Verification items for this drawing (mm, ordinates from the low corner). Round coordinates to 2 decimals unless told otherwise and drop trailing zeros. Loops run counter-clockwise (first coordinate to the right, second up) from the corner with the lowest first, then second, coordinate; pieces in that order, holes last. Notation, with made-up numbers: (-11, 40.5) - (22, 40.5) arc R12 cw to (22, 48.5) - close; hole circle Ø10 at (-20.75, 66). An arc over 180 degrees is marked (long way). Write item = value, one per line.
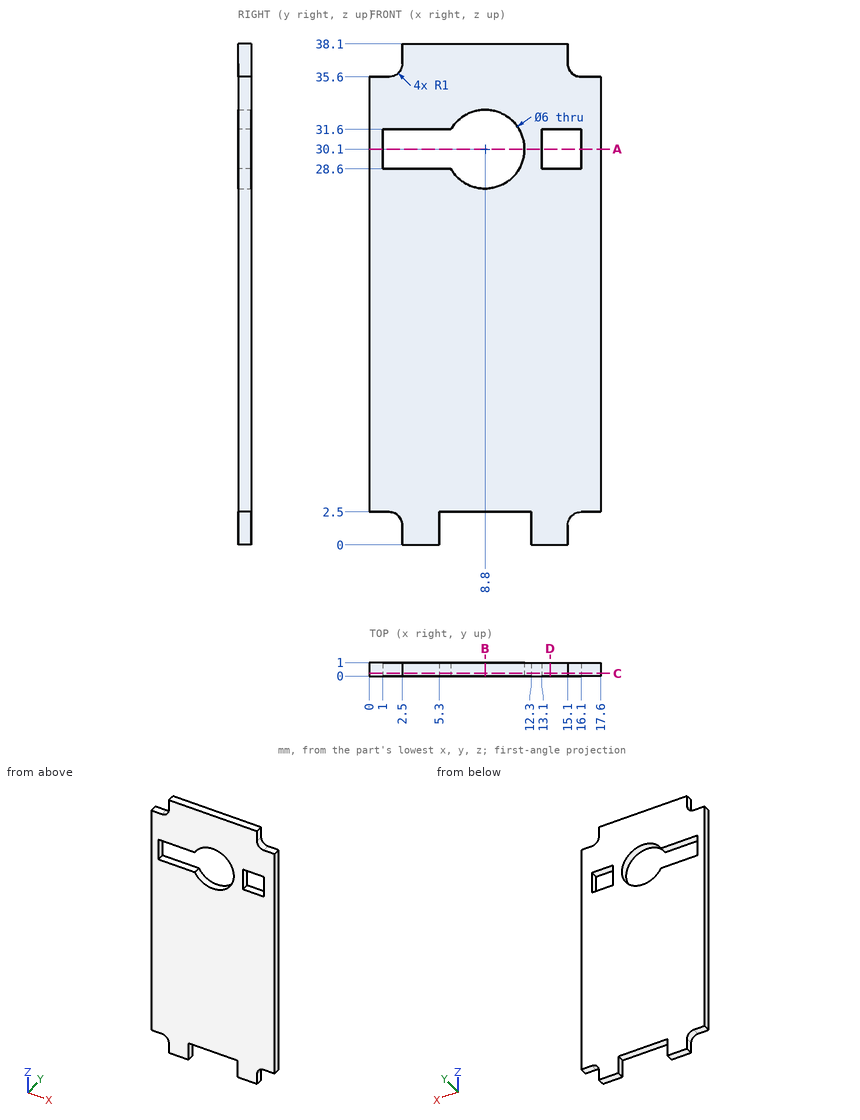
(1) Section check D-D (x = 13.75). Enter the section's corners in (y, z), then the cut area to 3 significant figures.
Answers follow:
outline = (0, 0) - (1, 0) - (1, 28.6) - (0, 28.6) - close; (0, 31.6) - (1, 31.6) - (1, 38.1) - (0, 38.1) - close
area = 35.1 mm²
(2) Section check C-C (y = 0.2). Enter the section's corners in (x, z).
Answers follow:
outline = (0, 2.5) - (1.5, 2.5) arc R1 cw to (2.5, 1.5) - (2.5, 0) - (5.3, 0) - (5.3, 2.5) - (12.3, 2.5) - (12.3, 0) - (15.1, 0) - (15.1, 1.5) arc R1 cw to (16.1, 2.5) - (17.6, 2.5) - (17.6, 35.6) - (16.1, 35.6) arc R1 cw to (15.1, 36.6) - (15.1, 38.1) - (2.5, 38.1) - (2.5, 36.6) arc R1 cw to (1.5, 35.6) - (0, 35.6) - close; hole (1, 28.6) - (6.2, 28.6) arc R3 ccw (long way) to (6.2, 31.6) - (1, 31.6) - close; hole (13.1, 28.6) - (16.1, 28.6) - (16.1, 31.6) - (13.1, 31.6) - close
(3) Section check B-B (x = 8.8). Enter the section's corners in (y, z), then the cut area to 3 significant figures.
Answers follow:
outline = (0, 2.5) - (1, 2.5) - (1, 27.1) - (0, 27.1) - close; (0, 33.1) - (1, 33.1) - (1, 38.1) - (0, 38.1) - close
area = 29.6 mm²
(4) Section check A-A (z = 30.1). Enter the section's corners in (x, y), then the cut area to 3 significant figures.
Answers follow:
outline = (0, 0) - (1, 0) - (1, 1) - (0, 1) - close; (11.8, 0) - (13.1, 0) - (13.1, 1) - (11.8, 1) - close; (16.1, 0) - (17.6, 0) - (17.6, 1) - (16.1, 1) - close
area = 3.80 mm²
(5) Scan lines: L1, parallel to X at y = 0.55, z = 30.1; L2, parallel to Z at x = 3.75, y = 0.4; L3, parallel to Z at x = 6, y = 0.7. Record each from-to range of solid material in increasing order. Write a range as [from, to].
Answers follow:
L1 = [0, 1], [11.8, 13.1], [16.1, 17.6]
L2 = [0, 28.6], [31.6, 38.1]
L3 = [2.5, 28.6], [31.6, 38.1]
(6) Gauge pin test, flat end, axial feed: pin 1 (0.5 mm diameter, centred on x = 0.5, y = 0.5, fed in from -Z). Record the tip position at first contact, or that the pin passes through.
Answers follow:
pin_1 = 2.5
